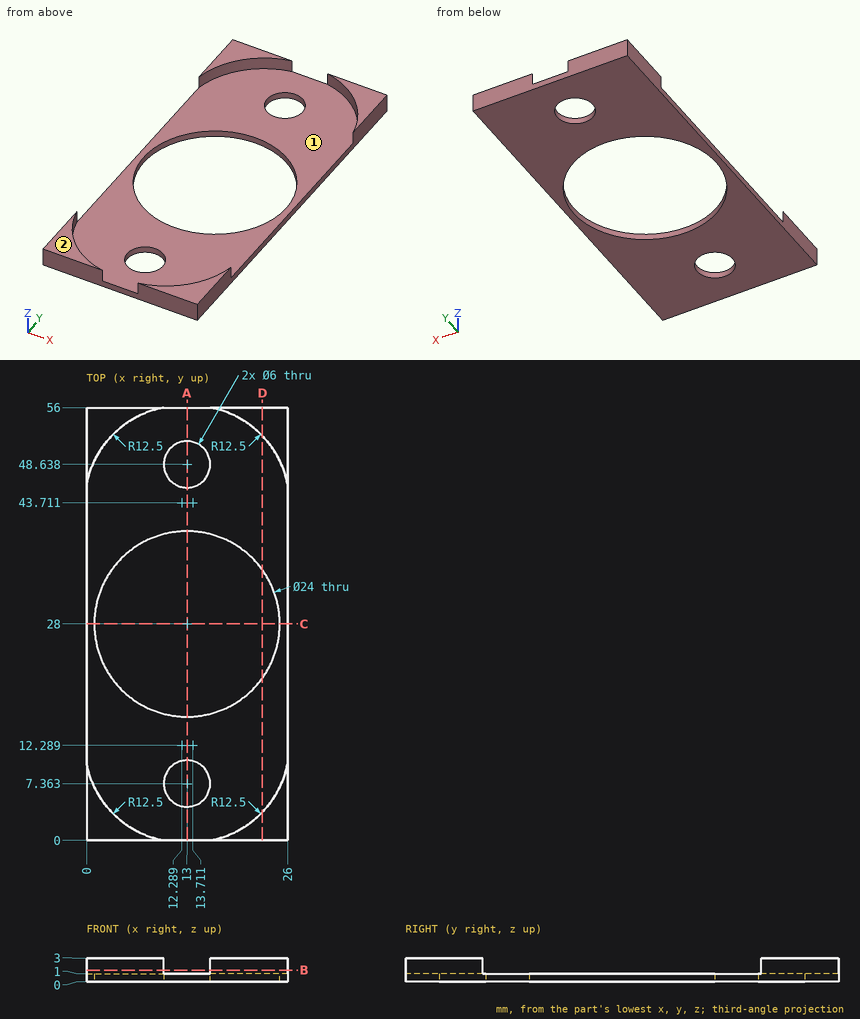
Design review of the part shown in the three views and the two pictorial views. Dimensions are in mm from the part's minimum x, y and z. Give positions to 0.01 mm unless a question says otherwise; leave off trailing zeros. Loops run counter-clockwise (first coordinate to the right, second up) from the corner with the lowest first, then second, coordinate; pieces in that order, holes last. Notation, with made-up numbers: M -35.5,-25.5 L -1.5,-25.5 A22 cw -1.5,-10.5 Z; hole C 7,1.5 d11. An arc over 180 degrees is marked long. Answer as a JSON object with one key per item and string values. Group by question number.
Q1. Insertion check: P1, Ø6, axis at x = 21, y = 20, coming from the +Z side; P2, Ø14.5, axis at x = 13, y = 28, coming from the +Z side; P3, Ø2, axis at x = 21, y = 17.5, coming from the -Z side. Each pin has a flat end and moves straight along its axis. Give the tip position at first contact, or say it passes through.
Q2. For probe 1 along Y at (x, z) = (13, 0.4); probe 2 along X at (y, z) = (7.5, 0.3); probe 3 along Z at (x, y) = (8, 50.5), list the stretches that pass through material, from the lowest coordinate up. Write a range as [from, to].
Q3. Add section B-B on z = 1.5. Give the boundary of the cut face in (x, y).
Q4. Mouldability with a two-part tool opening along Y and no side actions: class the marked faces 1 and 2 as +Y half, -Y half, draft (parallel to the pull), parting line (faces both ways), or undercut.
Q5. Add section A-A on x = 13. Give the boundary of the cut face in (y, z).
Q6. Add section D-D on x = 22.75. Give the boundary of the cut face in (y, z) (1 decimal).
Q7. Add section C-C on y = 28. Give the boundary of the cut face in (x, z).
Checked values:
{
 "1": {"P1": "z = 1", "P2": "through", "P3": "z = 0"},
 "2": {"probe 1": "[0, 4.36], [10.36, 16], [40, 45.64], [51.64, 56]", "probe 2": "[0, 10], [16, 26]", "probe 3": "[0, 1]"},
 "3": {"outline": "M 0,0 L 10,0 A12.5 cw 0,10 Z; M 0,46 A12.5 cw 10,56 L 0,56 Z; M 16,0 L 26,0 L 26,10 A12.5 cw Z; M 16,56 A12.5 cw 26,46 L 26,56 Z"},
 "4": {"face 1": "undercut", "face 2": "draft"},
 "5": {"outline": "M 0,0 L 4.36,0 L 4.36,1 L 0,1 Z; M 10.36,0 L 16,0 L 16,1 L 10.36,1 Z; M 40,0 L 45.64,0 L 45.64,1 L 40,1 Z; M 51.64,0 L 56,0 L 56,1 L 51.64,1 Z"},
 "6": {"outline": "M 0,0 L 21,0 L 21,1 L 3.7,1 L 3.7,3 L 0,3 Z; M 35,0 L 56,0 L 56,3 L 52.3,3 L 52.3,1 L 35,1 Z"},
 "7": {"outline": "M 0,0 L 1,0 L 1,1 L 0,1 Z; M 25,0 L 26,0 L 26,1 L 25,1 Z"}
}
